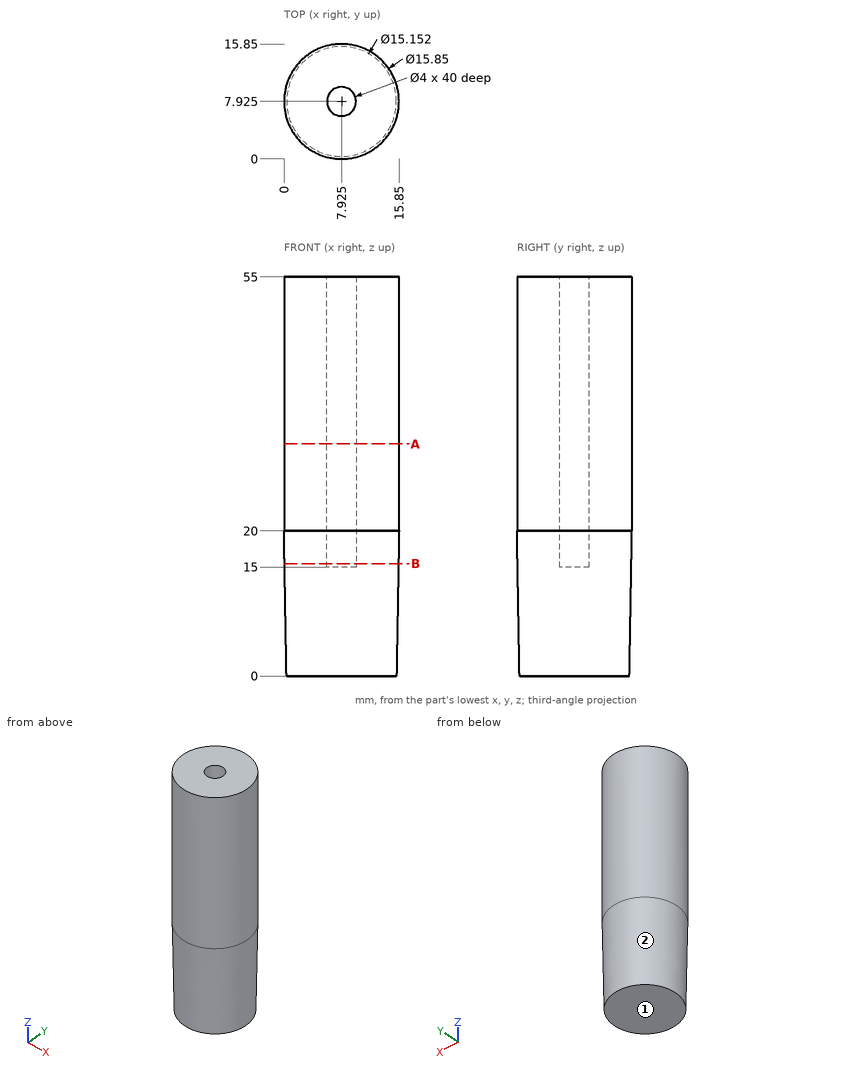
The figure shows three views and two pictorial views of one solid part (mm, origin at its lowest corner). Answer the questions. A direction names the side the tool comes from. Round coordinates to 2 decimals unless told otherwise and drop trailing zeros. Write each loop counter-clockwise with the first axis right and the second up, starting at its lowest first coordinate (ties: lowest second). Pieces come first, ordered by that corner, then holes. Notation, with made-up numbers: (2.5, -27.5) -> (22.5, -27.5) arc R16 ccw to (22.5, -8.5) -> close; hole circle Ø9 at (29, 66). An arc over 180 degrees is marked (long way). Answer as a JSON object with one key per item and string values. Group by question number.
Q1. Each of these flat-tipped pins is pushed along its axis until it touches: pin 1 Ø3 at (x, z) = (4.5, 12.5) entering from +Y; pin 2 Ø2 at (x, z) = (11, 21) entering from +Y; pin 3 Ø1.2 at (x, y) = (7.5, 7.5) entering from +Z. Where does it stop, or does it pass through?
Q2. Straight lines are drawn through the part: line 1 along Y through (x, z) = (9.5, 27); line 2 along Z through (x, y) = (7.5, 8.5); line 3 along X through (y, z) = (3.75, 13). For each, find the intervals that lie inside material, in ascending order.
Q3. Section A-A (z = 32) is taken. Write down the section's boundary in (x, y) (3 decimals).
Q4. Which of the six approach directions +Z, -Z, +X, -X, +Y, -Y give full straight-line access (tool end or side, diameter ignored) to the marked faces 1 and 2?
Q5. Section B-B (z = 15.5) is taken. Write down the section's boundary in (x, y) (1 decimal).
Check values:
{
 "1": {"pin 1": "y = 15.48", "pin 2": "y = 15.57", "pin 3": "z = 15"},
 "2": {"line 1": "0.16 to 6.69, 9.16 to 15.69", "line 2": "0 to 15", "line 3": "1.33 to 14.52"},
 "3": {"outline": "circle Ø15.85 at (7.925, 7.925); hole circle Ø4 at (7.925, 7.925)"},
 "4": {"face 1": "-Z, +X, -X, +Y, -Y", "face 2": "-Z"},
 "5": {"outline": "circle Ø15.7 at (7.9, 7.9); hole circle Ø4 at (7.9, 7.9)"}
}
